```python
from build123d import *

# Parameters (mm, degrees)
SKETCH2_R           = 6
BOSS_EXTRUDE1_DEPTH = 50
SKETCH3_R           = 9
BOSS_EXTRUDE2_DEPTH = 10
SKETCH4_R           = 6
BOSS_EXTRUDE3_DEPTH = 20
SKETCH6_W           = 4
SKETCH6_H           = 20
CUT_EXTRUDE1_DEPTH  = 2.2


with BuildPart() as part:
    # Sketch2 → Boss-Extrude1 (new body)
    with BuildSketch(Plane.XY):
        Circle(SKETCH2_R)
    extrude(amount=BOSS_EXTRUDE1_DEPTH)

    # Sketch3 → Boss-Extrude2 (add)
    with BuildSketch(Plane.XY.offset(50)):
        Circle(SKETCH3_R)
    extrude(amount=BOSS_EXTRUDE2_DEPTH)

    # Sketch4 → Boss-Extrude3 (add)
    with BuildSketch(Plane.XY.offset(60)):
        Circle(SKETCH4_R)
    extrude(amount=BOSS_EXTRUDE3_DEPTH)

    # Sketch6 → Cut-Extrude1 (cut)
    with BuildSketch(Plane(origin=(0, 6, 0), x_dir=(1, 0, 0), z_dir=(0, 1, 0))):
        with Locations((0, -30)):
            Rectangle(SKETCH6_W, SKETCH6_H)
    extrude(amount=-CUT_EXTRUDE1_DEPTH, mode=Mode.SUBTRACT)


solid = part.part
```
Work out the finished part from the listing and answer in its coordinate system (mm). A direction names the side the tool comes from. Give positions to 0.01 mm unless a question says otherwise; leave off trailing zeros. Loops run counter-clockwise (first coordinate to the right, second up) from the corner with the lowest first, then second, coordinate; pieces in that order, holes last. Notation, with made-up numbers: (15.25, 69) -> (36.25, 69) arc R25 ccw to (36.25, 105) -> close; hole circle Ø1 at (-25, 45.5). An arc over 180 degrees is marked (long way). Use CSV: the item, a comma, the result in double quotes.
1. A tool of negligible diameter and unlimited length cuts with its end or side. For faces 4 (the flat face through (0, 0, 80)), 5 (the flat face through (0, 5, 20)), 6 (the flat face through (2, -6, 50)), 7 (the cylindrical face through (-6, 0, 70)), 8 (the cylindrical face through (-1.172, 8.923, 54.93)), from which of +Z, -Z, +X, -X, +Y, -Y can it reach the whole face along a straight path? Write none if from no direction.
Found:
face 4,"+Z, +X, -X, +Y, -Y"
face 5,"+Y"
face 6,"-Z"
face 7,"+Z"
face 8,"+Z, -Z"
2. The part is cut by section D-D (x = -4.5). Write down the section's boundary in (y, z).
Found:
outline,"(-7.79, 50) -> (-3.97, 50) -> (-3.97, 0) -> (3.97, 0) -> (3.97, 50) -> (7.79, 50) -> (7.79, 60) -> (3.97, 60) -> (3.97, 80) -> (-3.97, 80) -> (-3.97, 60) -> (-7.79, 60) -> close"
3. The mould has two halves that part along X. Classify faces 1 (the flat face through (2, -6, 60)), 2 (the flat face through (2, 5, 30)), 3 (the cylindrical face through (-1.301, -5.857, 24.65)): +X half, -X half, draft (parallel to the pull), parting line (faces both ways), or undercut.
Found:
face 1,"draft"
face 2,"undercut"
face 3,"parting line"
4. Flat-ended cylindrical pins translate along their axes: pin 1 Ø1 at (x, z) = (5, 44) entering from +Y; pin 2 Ø1.5 at (x, z) = (-3, 19.5) entering from -Y; pin 3 Ø1 at (y, z) = (-1, 17.5) entering from +X. Find the tip coordinate at first contact, or state that the pin passes through.
Found:
pin 1,"y = 3.97"
pin 2,"y = -5.56"
pin 3,"x = 5.98"
5. The part is cut by section A-A (x = 0). Write down the section's boundary in (y, z).
Found:
outline,"(-9, 50) -> (-6, 50) -> (-6, 0) -> (6, 0) -> (6, 20) -> (3.8, 20) -> (3.8, 40) -> (6, 40) -> (6, 50) -> (9, 50) -> (9, 60) -> (6, 60) -> (6, 80) -> (-6, 80) -> (-6, 60) -> (-9, 60) -> close"
6. The part is cut by section C-C (z = 69). Write down the section's boundary in (x, y), then the cut area to 3 significant figures.
Found:
outline,"circle Ø12 at (0, 0)"
area,"113 mm^2"
7. Straight lines are drawn through the part: line 1 (Z direction, x = -4.5, y = -5.5); line 2 (X direction, y = -0.25, z = 33.5); line 3 (Y direction, x = -5.25, z = 24). For each, find the intervals that lie inside material, in ascending order.
Found:
line 1,"50 to 60"
line 2,"-5.99 to 5.99"
line 3,"-2.9 to 2.9"
8. The part is cut by section B-B (y = 0). Write down the section's boundary in (x, z), then the cut area to 3 significant figures.
Found:
outline,"(-9, 50) -> (-6, 50) -> (-6, 0) -> (6, 0) -> (6, 50) -> (9, 50) -> (9, 60) -> (6, 60) -> (6, 80) -> (-6, 80) -> (-6, 60) -> (-9, 60) -> close"
area,"1,020 mm^2"
